Build history of the part. All positions in model axes, mm. Face numbers are marked on the shaded views. A direction names the side the tool comes from. Give positions to 0.01 mm unless a question says otherwise; leave off trailing zeros. Loops run counter-clockwise (first coordinate to the right, second up) from the corner with the lowest first, then second, coordinate; pieces in that order, holes last. Notation, with made-up numbers: M -10,44 L 48,44 A19 cw 48,58 Z; hole C 30.25,-22.75 d8. An arc over 180 degrees is marked long. Answer in a Markdown table with one row per item. Add a question column.
```python
from build123d import *

# Parameters (mm, degrees)
S_LIMITSWITCH_W = 40
S_LIMITSWITCH_H = 17
PAD024_DEPTH    = 2
SKETCH053_W     = 7.5
SKETCH053_H     = 12.5
PAD025_DEPTH    = 5
SKETCH054_R     = 1.5
POCKET029_DEPTH = 5


with BuildPart() as part:
    # S_LimitSwitch → Pad024 (new body)
    with BuildSketch(Plane.XY):
        Rectangle(S_LIMITSWITCH_W, S_LIMITSWITCH_H)
    extrude(amount=PAD024_DEPTH)

    # Sketch053 → Pad025 (join)
    with BuildSketch(Plane.XY.offset(2)):
        Polygon((13.3, 8), (13.3, 1.3), (0.5, 1.3), (0.5, 8), (1.5, 8), (16.5, 12), (17, 12), (2, 8), align=None)
        with Locations((-13.25, 0.25)):
            Rectangle(SKETCH053_W, SKETCH053_H)
    extrude(amount=PAD025_DEPTH)

    # Sketch054 → Pocket029 (cut)
    with BuildSketch(Plane.XY.offset(3)):
        with Locations((16.5, 5.8)):
            Circle(SKETCH054_R)
        with Locations((-2.75, 5.8)):
            Circle(SKETCH054_R)
    extrude(amount=-POCKET029_DEPTH, mode=Mode.SUBTRACT)


solid = part.part
```
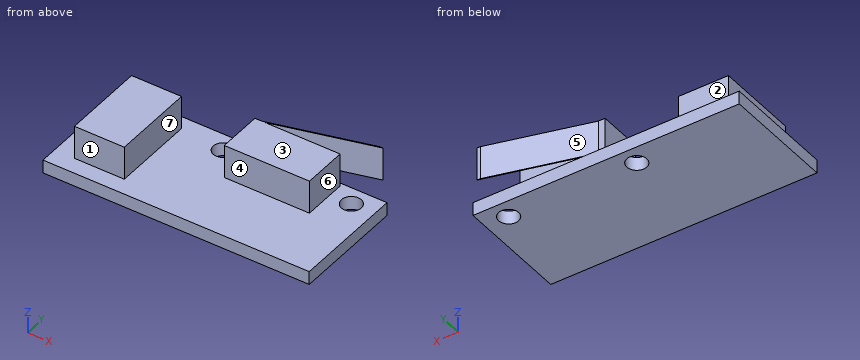
(1) Slice it at C-C, the plane z = 3. Give the cut face in (x, y), then the cut area to 3 significant figures.
(2) Tool access for the marked faces 1, 2, 3 and 4: list every direction of +Z, -Z, +X, -X, +Y, -Y with a clear straight run to the whole face (end or side of a thin tool).
(3) Slice it at A-A, the plane y = 5.8. Give the cut face in (x, z), then the cut area to 4 significant figures.
(4) Pull direction X, two halves, no side cores. Call the marked faces 5, 6 and 7: +X half, -X half, draft (parallel to the pull), parting line (faces both ways), or undercut.
(5) Slice it at B-B, the plane x = -2.75. Give the cut face in (y, z), then the cut area to 3 significant figures.
(6) Slice it at D-D, the plane y = 1.75. Give the cut face in (x, z).
(7) Pin check, flat tips, straight feed: pin 1 (4 mm diameter, centred on y = 3.5, z = 5, fed in from +X); pin 2 (4 mm diameter, centred on x = -15, z = 5.5, fed in from +Y); pin 3 (1.1 mm diameter, centred on x = 1, z = 5, fed in from +Y). Stop position of each tip, or through.
(8) Wall check: line 1 (Y direction, x = -2.75, z = 1.15); line 2 (X direction, y = 6, z = 2.5); line 3 (Z direction, x = -13.5, y = 8). Give the ranges that are in metal, low to high.
Solution:
| question | item | result |
|---|---|---|
| 1 | outline | M -17,-6 L -9.5,-6 L -9.5,6.5 L -17,6.5 Z; M 0.5,1.3 L 13.3,1.3 L 13.3,8 L 2,8 L 17,12 L 16.5,12 L 1.5,8 L 0.5,8 Z |
| 1 | area | 182 mm^2 |
| 2 | face 1 | +Z, +X, -X, -Y |
| 2 | face 2 | +Z, -X, +Y |
| 2 | face 3 | +Z, +X, -X, +Y, -Y |
| 2 | face 4 | +Z, +X, -Y |
| 3 | outline | M -20,0 L -4.25,0 L -4.25,2 L -9.5,2 L -9.5,7 L -17,7 L -17,2 L -20,2 Z; M -1.25,0 L 15,0 L 15,2 L 13.3,2 L 13.3,7 L 0.5,7 L 0.5,2 L -1.25,2 Z; M 18,0 L 20,0 L 20,2 L 18,2 Z |
| 3 | area | 169.5 mm^2 |
| 4 | face 5 | -X half |
| 4 | face 6 | +X half |
| 4 | face 7 | undercut |
| 5 | outline | M -8.5,0 L 4.3,0 L 4.3,2 L -8.5,2 Z; M 7.3,0 L 8.5,0 L 8.5,2 L 7.3,2 Z |
| 5 | area | 28.0 mm^2 |
| 6 | outline | M -20,0 L 20,0 L 20,2 L 13.3,2 L 13.3,7 L 0.5,7 L 0.5,2 L -9.5,2 L -9.5,7 L -17,7 L -17,2 L -20,2 Z |
| 7 | pin 1 | x = 13.3 |
| 7 | pin 2 | y = 6.5 |
| 7 | pin 3 | y = 8.01 |
| 8 | line 1 | -8.5 to 4.3, 7.3 to 8.5 |
| 8 | line 2 | -17 to -9.5, 0.5 to 13.3 |
| 8 | line 3 | 0 to 2 |
